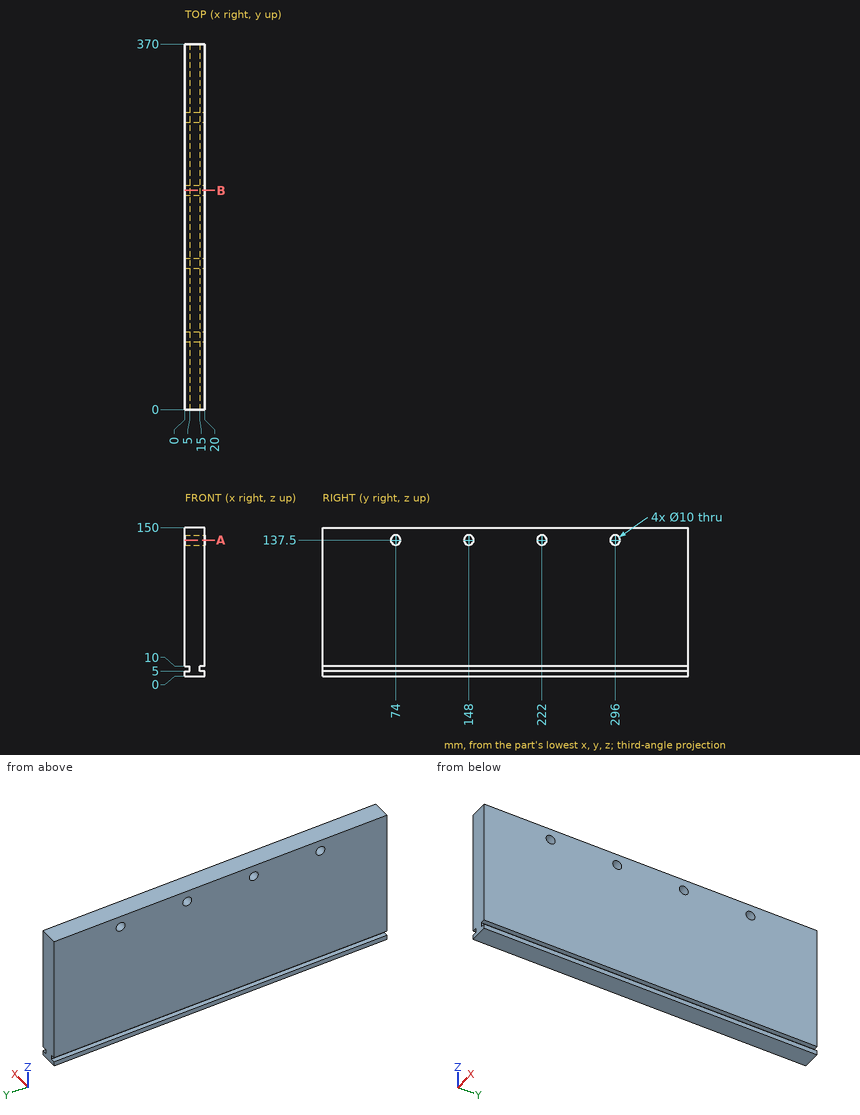
The drawing under review shows one solid part. Ordinate dimensions are in mm from its lowest x, y, z. Round coordinates to 2 decimals unless told otherwise and drop trailing zeros. Order: outer loops, then holes, each group sorted by start corner. A loop starts at its lowest first (then second) coordinate and runs counter-clockwise, first axis right, second up. Notation, with made-up numbers: (81, 45) -> (126, 45) arc R27 ccw to (126, 77) -> close; hole circle Ø10 at (32.25, 8). An arc over 180 degrees is marked (long way). Use a Markdown table: item, result.
Item 1: For pin 1 (11.5 mm diameter, centred on y = 222, z = 137.5, fed in from +X); pin 2 (6 mm diameter, centred on y = 148, z = 137.5, fed in from -X), all flat-tipped, find the tip position at first contact; note any pin that passes through.
Resolved:
| item | result |
|---|---|
| pin 1 | stops at x = 20 |
| pin 2 | passes through |
Item 2: Take a section at B-B (y = 222). State the section outline as (x, z) points.
Resolved:
| item | result |
|---|---|
| outline | (0, 0) -> (20, 0) -> (20, 5) -> (15, 5) -> (15, 10) -> (20, 10) -> (20, 132.5) -> (0, 132.5) -> (0, 10) -> (5, 10) -> (5, 5) -> (0, 5) -> close; (0, 142.5) -> (20, 142.5) -> (20, 150) -> (0, 150) -> close |
Item 3: Take a section at A-A (z = 137.5). State the section outline as (x, y) points, plus the area to 3 significant figures.
Resolved:
| item | result |
|---|---|
| outline | (0, 0) -> (20, 0) -> (20, 69) -> (0, 69) -> close; (0, 79) -> (20, 79) -> (20, 143) -> (0, 143) -> close; (0, 153) -> (20, 153) -> (20, 217) -> (0, 217) -> close; (0, 227) -> (20, 227) -> (20, 291) -> (0, 291) -> close; (0, 301) -> (20, 301) -> (20, 370) -> (0, 370) -> close |
| area | 6,600 mm² |
Item 4: For line 1 along Y through (x, z) = (8.25, 137.5); line 2 along Y through (x, z) = (12, 134.5); line 3 along Z through (x, y) = (3.75, 60), list the stretches that pass through material, from the lowest coordinate up. Write a range as [from, to].
Resolved:
| item | result |
|---|---|
| line 1 | y = [0, 69], [79, 143], [153, 217], [227, 291], [301, 370] |
| line 2 | y = [0, 70], [78, 144], [152, 218], [226, 292], [300, 370] |
| line 3 | z = [0, 5], [10, 150] |
